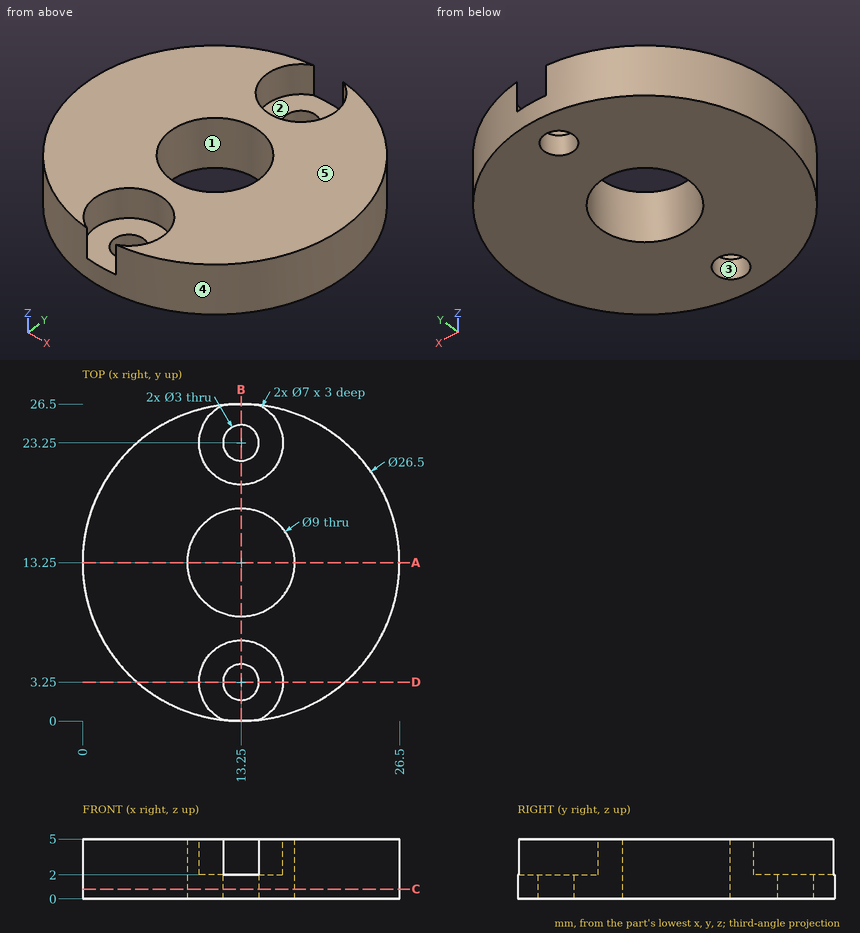
Verification items for this drawing (mm, ordinates from the low corner). A direction names the side the tool comes from. Round coordinates to 2 decimals unless told otherwise and drop trailing zeros. Write each loop counter-clockwise with the first axis right and the second up, starting at its lowest first coordinate (ties: lowest second). Pieces come first, ordered by that corner, then holes. Notation, with made-up numbers: M 22,30.25 L 34,30.25 A21 ccw 34,43.25 Z; hole C 37.25,16 d8. An arc over 180 degrees is marked long. Write item = value, one per line. Start each with the question number.
1. Section check A-A, the plane y = 13.25. Record the cut outline in (x, z).
2. Tool access check on the marked faces 1 and 2. Record the directions out of +Z, -Z, +X, -X, +Y, -Y that give a thin tool (end or side, any length) a straight path to the whole face; none if there is none.
3. Section check D-D, the plane y = 3.25. Record the cut outline in (x, z).
4. Section check B-B, the plane x = 13.25. Record the cut outline in (y, z).
5. Release check for a two-part mould opening along X. For the marked faces 3, 4 and 5 record: pulls with the +X half, pulls with the -X half, needs draft (parallel to the pull), parting line crosses it, or undercut.
6. Section check C-C, the plane z = 0.8. Record the cut outline in (x, y).
7. Scan lines: line 1 (Y direction, x = 13.25, z = 1.1); line 2 (Y direction, x = 11, z = 1.5); line 3 (Y direction, x = 13, z = 2.6). Record each from-to range of solid material in increasing order. Write a range as [from, to].
8. Gauge pin test, flat ends, axial feed: pin 1 (4 mm diameter, centred on x = 13.25, y = 23.25, fed in from +Z); pin 2 (5 mm diameter, centred on x = 13.25, y = 23.25, fed in from -Z). Record the tip position at first contact, or that the pin passes through.
Results found:
q1.outline = M 0,0 L 8.75,0 L 8.75,5 L 0,5 Z; M 17.75,0 L 26.5,0 L 26.5,5 L 17.75,5 Z
q2.face_1 = +Z, -Z
q2.face_2 = +Z
q3.outline = M 4.56,0 L 11.75,0 L 11.75,2 L 9.75,2 L 9.75,5 L 4.56,5 Z; M 14.75,0 L 21.94,0 L 21.94,5 L 16.75,5 L 16.75,2 L 14.75,2 Z
q4.outline = M 0,0 L 1.75,0 L 1.75,2 L 0,2 Z; M 4.75,0 L 8.75,0 L 8.75,5 L 6.75,5 L 6.75,2 L 4.75,2 Z; M 17.75,0 L 21.75,0 L 21.75,2 L 19.75,2 L 19.75,5 L 17.75,5 Z; M 24.75,0 L 26.5,0 L 26.5,2 L 24.75,2 Z
q5.face_3 = undercut
q5.face_4 = parting line crosses it
q5.face_5 = needs draft
q6.outline = C 13.25,13.25 d26.5; hole C 13.25,13.25 d9; hole C 13.25,3.25 d3; hole C 13.25,23.25 d3
q7.line_1 = [0, 1.75], [4.75, 8.75], [17.75, 21.75], [24.75, 26.5]
q7.line_2 = [0.19, 9.35], [17.15, 26.31]
q7.line_3 = [6.74, 8.76], [17.74, 19.76]
q8.pin_1 = 2
q8.pin_2 = 0
